from build123d import *

# Parameters (mm, degrees)
SKETCH1_W           = 32
SKETCH1_H           = 53
SKETCH1_R           = 1.1
BOSS_EXTRUDE1_DEPTH = 2.5
CUT_EXTRUDE2_DEPTH  = 32.056400307
FILLET1_R           = 2


with BuildPart() as part:
    # Sketch1 → Boss-Extrude1 (new body)
    with BuildSketch(Plane.XY):
        Rectangle(SKETCH1_W, SKETCH1_H)
        with Locations((-12, 23.5)):
            Circle(SKETCH1_R, mode=Mode.SUBTRACT)
        with Locations((12, -23.5)):
            Circle(SKETCH1_R, mode=Mode.SUBTRACT)
        with Locations((12, 23.5)):
            Circle(SKETCH1_R, mode=Mode.SUBTRACT)
        with Locations((-12, -23.5)):
            Circle(SKETCH1_R, mode=Mode.SUBTRACT)
    extrude(amount=BOSS_EXTRUDE1_DEPTH)

    # Sketch4 → Cut-Extrude2 (cut, through all)
    with BuildSketch(Plane.XY.offset(2.5)):
        with BuildLine():
            Line((-8, 18), (8, 18))
            ThreePointArc((8, 18), (10.5, 15.5), (8, 13))
            Line((8, 13), (-8, 13))
            ThreePointArc((-8, 13), (-10.5, 15.5), (-8, 18))
        make_face()
        with BuildLine():
            Line((-8, 2.666666667), (8, 2.666666667))
            ThreePointArc((8, 2.666666667), (10.5, 5.166666667), (8, 7.666666667))
            Line((8, 7.666666667), (-8, 7.666666667))
            ThreePointArc((-8, 7.666666667), (-10.5, 5.166666667), (-8, 2.666666667))
        make_face()
        with BuildLine():
            Line((-8, -7.666666667), (8, -7.666666667))
            ThreePointArc((8, -7.666666667), (10.5, -5.166666667), (8, -2.666666667))
            Line((8, -2.666666667), (-8, -2.666666667))
            ThreePointArc((-8, -2.666666667), (-10.5, -5.166666667), (-8, -7.666666667))
        make_face()
        with BuildLine():
            Line((-8, -18), (8, -18))
            ThreePointArc((8, -18), (10.5, -15.5), (8, -13))
            Line((8, -13), (-8, -13))
            ThreePointArc((-8, -13), (-10.5, -15.5), (-8, -18))
        make_face()
    extrude(amount=-CUT_EXTRUDE2_DEPTH, mode=Mode.SUBTRACT)

    # Fillet1
    fillet1_edges = [part.edges().sort_by_distance(p)[0] for p in [
        (16, -26.5, 1.25),
        (-16, -26.5, 1.25),
        (-16, 26.5, 1.25),
        (16, 26.5, 1.25),
    ]]
    fillet(fillet1_edges, radius=FILLET1_R)


solid = part.part
For this review, take the finished solid that the model builds, in its own axes (mm). A direction names the side the tool comes from. Round coordinates to 2 decimals unless told otherwise and drop trailing zeros. Order: outer loops, then holes, each group sorted by start corner. A loop starts at its lowest first (then second) coordinate and runs counter-clockwise, first axis right, second up. Notation, with made-up numbers: (-8, 55.25) -> (46, 55.25) arc R27 cw to (46, 82.25) -> close; hole circle Ø3 at (57, 58). An arc over 180 degrees is marked (long way). Write item = value, one per line. Start each with the question number.
1) The part is to be moulded in two halves that separate along X. For faces 1 (the face through (0, 0, 0)), 2 (the face through (15.4, -25.93, 1.27)), 3 (the face through (-10.5, 15.4, 1.3)), say which applies: +X half, -X half, draft (parallel to the pull), parting line (faces both ways), or undercut.
2) Take a section at A-A on y = 23.5. State the section outline as (x, z) points.
3) Insertion check: pin 1 (12 mm diameter, centred on x = -2.5, y = -4, fed in from -Z); pin 2 (1.8 mm diameter, centred on x = 12, y = -23.5, fed in from +Z). Each pin has a flat end and moves straight along its axis. Give the tip position at first contact, or say it passes through.
4) Take a section at D-D on y = -15.5. State the section outline as (x, z) points.
5) Take a section at B-B on x = -12. State the section outline as (y, z) points.
6) Tool access review of faces 4 (the face through (15.4, 25.93, 1.27)), 5 (the face through (-10.5, -15.4, 1.3)): name each direction out of +Z, -Z, +X, -X, +Y, -Y from which nothing blocks a thin tool from reaching the whole face with its end or side.
7) Take a section at C-C on x = 7. State the section outline as (y, z) points.
8) To check wall thickness, follow line 1 (Y direction, x = -12, z = 1.5); line 2 (Y direction, x = -7, z = 1.6); line 3 (X direction, y = -15.5, z = 1.85). State the ranges of each line that lie inside material, in increasing order. Write a range as from..to.
Verdict:
q1.face_1 = draft
q1.face_2 = +X half
q1.face_3 = undercut
q2.outline = (-16, 0) -> (-13.1, 0) -> (-13.1, 2.5) -> (-16, 2.5) -> close; (-10.9, 0) -> (10.9, 0) -> (10.9, 2.5) -> (-10.9, 2.5) -> close; (13.1, 0) -> (16, 0) -> (16, 2.5) -> (13.1, 2.5) -> close
q3.pin_1 = 0
q3.pin_2 = through
q4.outline = (-16, 0) -> (-10.5, 0) -> (-10.5, 2.5) -> (-16, 2.5) -> close; (10.5, 0) -> (16, 0) -> (16, 2.5) -> (10.5, 2.5) -> close
q5.outline = (-26.5, 0) -> (-24.6, 0) -> (-24.6, 2.5) -> (-26.5, 2.5) -> close; (-22.4, 0) -> (22.4, 0) -> (22.4, 2.5) -> (-22.4, 2.5) -> close; (24.6, 0) -> (26.5, 0) -> (26.5, 2.5) -> (24.6, 2.5) -> close
q6.face_4 = +Z, -Z, +X, +Y
q6.face_5 = +Z, -Z
q7.outline = (-26.5, 0) -> (-18, 0) -> (-18, 2.5) -> (-26.5, 2.5) -> close; (-13, 0) -> (-7.67, 0) -> (-7.67, 2.5) -> (-13, 2.5) -> close; (-2.67, 0) -> (2.67, 0) -> (2.67, 2.5) -> (-2.67, 2.5) -> close; (7.67, 0) -> (13, 0) -> (13, 2.5) -> (7.67, 2.5) -> close; (18, 0) -> (26.5, 0) -> (26.5, 2.5) -> (18, 2.5) -> close
q8.line_1 = -26.5..-24.6, -22.4..22.4, 24.6..26.5
q8.line_2 = -26.5..-18, -13..-7.67, -2.67..2.67, 7.67..13, 18..26.5
q8.line_3 = -16..-10.5, 10.5..16
